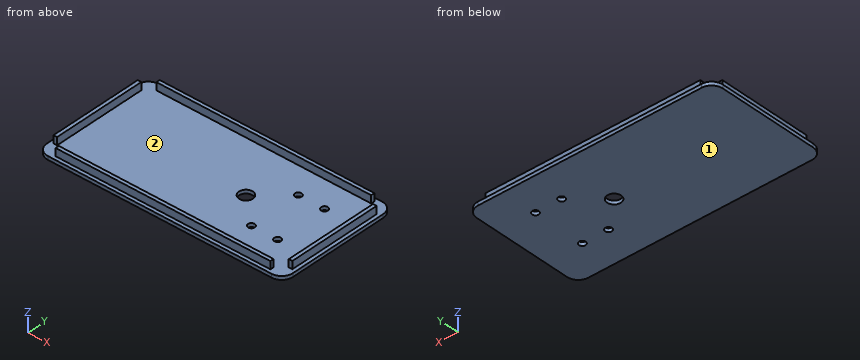
```python
from build123d import *

# Parameters (mm, degrees)
F0_W     = 110
F0_H     = 55
F1_DEPTH = 1.6
F2_R     = 1.5
F2_R_2   = 3.1
F3_DEPTH = 1.6
F2_W     = 96
F2_H     = 1.6
F2_W_2   = 1.6
F2_H_2   = 42
F4_DEPTH = 3.4
F5_R     = 5


with BuildPart() as f1:
    # F0 (on Top) → F1 (new body)
    with BuildSketch(Plane.XY):
        Rectangle(F0_W, F0_H)
    extrude(amount=F1_DEPTH)

    # F2 (on face) → F3 (cut, through all)
    with BuildSketch(Plane.XY.offset(1.6)):
        with Locations((26.762206, 11.680291)):
            Circle(F2_R)
        with Locations((38.488474, 11.680291)):
            Circle(F2_R)
        with Locations((26.762206, -11.680291)):
            Circle(F2_R)
        with Locations((38.488474, -11.680291)):
            Circle(F2_R)
        with Locations((13.829022, 0)):
            Circle(F2_R_2)
    extrude(amount=-F3_DEPTH, mode=Mode.SUBTRACT)

    # F2 (on face) → F4 (join)
    with BuildSketch(Plane.XY.offset(1.6)):
        with Locations((0, 25.1)):
            Rectangle(F2_W, F2_H)
        with Locations((-52.6, 0)):
            Rectangle(F2_W_2, F2_H_2)
        with Locations((0, -25.1)):
            Rectangle(F2_W, F2_H)
        with Locations((52.6, 0)):
            Rectangle(F2_W_2, F2_H_2)
    extrude(amount=F4_DEPTH)

    # F5
    f5_edges = [f1.edges().sort_by_distance(p)[0] for p in [
        (55, -27.5, 0.8),
        (-55, -27.5, 0.8),
        (55, 27.5, 0.8),
        (-55, 27.5, 0.8),
    ]]
    fillet(f5_edges, radius=F5_R)


solid = f1.part
```
Source: CAD feature listing. Evaluate the final solid. Frame: model axes, mm. Face numbers are marked on the shaded views. Give positions to 0.01 mm unless a question says otherwise; leave off trailing zeros. Write each loop counter-clockwise with the first axis right and the second up, starting at its lowest first coordinate (ties: lowest second). Pieces come first, ordered by that corner, then holes. Notation, with made-up numbers: (-8, 52.25) - (41, 52.25) arc R27 ccw to (41, 84.25) - close; hole circle Ø7 at (-20, 11). An arc over 180 degrees is marked (long way). One line per item, written item: value. Start each with the question number.
Q1. Section query C-C, the plane y = 19. Return the cut outline in (x, z).
Q2. Section query B-B, the plane y = 0. Return the cut outline in (x, z).
Q3. Section query D-D, the plane x = 18.5. Return the cut outline in (y, z).
Q4. Section query A-A, the plane z = 2.9. Return the cut outline in (x, y).
Q5. Material intervals for probe 1 along Y at (x, z) = (41.5, 4.2); probe 2 along X at (y, z) = (-1.5, 4.5); probe 3 along Z at (x, y) = (19.5, 12), sorted ascending. Write a range as from..to.
Q6. First-contact query: pin 1 Ø2.5 at (x, y) = (38.49, 11.68) entering from +Z; pin 2 Ø3 at (x, z) = (29, 3.5) entering from -Y; pin 3 Ø1.3 at (x, z) = (-52.5, 2.5) entering from -Y; pin 4 Ø0.5 at (y, z) = (-25.5, 3) entering from +X. Flat tips, straight axial feed; report the tip coordinate or a pass-through.
Q7. Draft query along X for the marked faces 1 and 2. Return one class per face: +X half, -X half, draft (parallel to the pull), parting line (faces both ways), or undercut.
Answer:
1. outline: (-55, 0) - (55, 0) - (55, 1.6) - (53.4, 1.6) - (53.4, 5) - (51.8, 5) - (51.8, 1.6) - (-51.8, 1.6) - (-51.8, 5) - (-53.4, 5) - (-53.4, 1.6) - (-55, 1.6) - close
2. outline: (-55, 0) - (10.73, 0) - (10.73, 1.6) - (-51.8, 1.6) - (-51.8, 5) - (-53.4, 5) - (-53.4, 1.6) - (-55, 1.6) - close; (16.93, 0) - (55, 0) - (55, 1.6) - (53.4, 1.6) - (53.4, 5) - (51.8, 5) - (51.8, 1.6) - (16.93, 1.6) - close
3. outline: (-27.5, 0) - (27.5, 0) - (27.5, 1.6) - (25.9, 1.6) - (25.9, 5) - (24.3, 5) - (24.3, 1.6) - (-24.3, 1.6) - (-24.3, 5) - (-25.9, 5) - (-25.9, 1.6) - (-27.5, 1.6) - close
4. outline: (-53.4, -21) - (-51.8, -21) - (-51.8, 21) - (-53.4, 21) - close; (-48, -25.9) - (48, -25.9) - (48, -24.3) - (-48, -24.3) - close; (-48, 24.3) - (48, 24.3) - (48, 25.9) - (-48, 25.9) - close; (51.8, -21) - (53.4, -21) - (53.4, 21) - (51.8, 21) - close
5. probe 1: y = -25.9..-24.3, 24.3..25.9
5. probe 2: x = -53.4..-51.8, 51.8..53.4
5. probe 3: z = 0..1.6
6. pin 1: passes through
6. pin 2: stops at y = -25.9
6. pin 3: stops at y = -21
6. pin 4: stops at x = 48
7. face 1: draft
7. face 2: undercut
